Geometry check sheet. Reference: the model listing, model coordinates, mm. A direction names the side the tool comes from. Give positions to 0.01 mm unless a question says otherwise; leave off trailing zeros. Write each loop counter-clockwise with the first axis right and the second up, starting at its lowest first coordinate (ties: lowest second). Pieces come first, ordered by that corner, then holes. Notation, with made-up numbers: M 39,41.25 L 87,41.25 A19 ccw 87,77.25 Z; hole C 58.5,49.25 d9. An arc over 180 degrees is marked long. Use one line per item in the form item = value. Start each with the question number.
```python
from build123d import *

# Parameters (mm, degrees)
SKETCH1_W           = 22
SKETCH1_H           = 22
BOSS_EXTRUDE1_DEPTH = 17
SKETCH5_R           = 7
BOSS_EXTRUDE4_DEPTH = 3
SKETCH6_R           = 10
BOSS_EXTRUDE5_DEPTH = 13
SKETCH7_R           = 5.5
CUT_EXTRUDE1_DEPTH  = 37.482872694
SKETCH8_R           = 3.25
CUT_EXTRUDE2_DEPTH  = 46.5


with BuildPart() as part:
    # Sketch1 → Boss-Extrude1 (new body)
    with BuildSketch(Plane.XY):
        Rectangle(SKETCH1_W, SKETCH1_H)
    extrude(amount=BOSS_EXTRUDE1_DEPTH)

    # Sketch5 → Boss-Extrude4 (add)
    with BuildSketch(Plane.XY):
        Circle(SKETCH5_R)
    extrude(amount=-BOSS_EXTRUDE4_DEPTH)

    # Sketch6 → Boss-Extrude5 (add)
    with BuildSketch(Plane(origin=(0, 0, -3), x_dir=(-1, 0, 0), z_dir=(0, 0, -1))):
        Circle(SKETCH6_R)
    extrude(amount=BOSS_EXTRUDE5_DEPTH)

    # Sketch7 → Cut-Extrude1 (cut, through all)
    with BuildSketch(Plane.XY.offset(17)):
        Circle(SKETCH7_R)
    extrude(amount=-CUT_EXTRUDE1_DEPTH, mode=Mode.SUBTRACT)

    # Sketch8 → Cut-Extrude2 (cut, symmetric)
    with BuildSketch(Plane(origin=(11, 0, 0), x_dir=(0, 0, -1), z_dir=(1, 0, 0))):
        with Locations(Location((-8.5, 0, 0), (0, 0, 90))):
            Circle(SKETCH8_R)
    extrude(amount=CUT_EXTRUDE2_DEPTH, both=True, mode=Mode.SUBTRACT)


solid = part.part
```
(1) Sectioned sample at A-A, the plane x = 0. Record the boundary of the cut face in (y, z), plus the area to 3 significant figures.
(2) Sectioned sample at B-B, the plane z = 8.5. Record the boundary of the cut face in (x, y).
(3) Tool access check on faces 5 (the cylindrical face through (2.17, -9.76, -9.41)), 6 (the cylindrical face through (6.466, -2.681, -1.479)), 7 (the flat face through (11, -3, 6)). Record the directions out of +Z, -Z, +X, -X, +Y, -Y that give a thin tool (end or side, any length) a straight path to the whole face; none if there is none.
(4) Sectioned sample at C-C, the plane y = 0. Record the boundary of the cut face in (x, z).
(5) Depth check by flat-ended pin: pin 1 (4 mm diameter, centred on y = -3, z = -5, fed in from -X); pin 2 (5 mm diameter, centred on x = 6, z = -5, fed in from +Y); pin 3 (10 mm diameter, centred on y = 1, z = -5.5, fed in from -X). Enter the tip coordinate at first touch or a pass-through.
(6) Thickness scan on probe 1 along Z at (x, y) = (-7.5, 0); probe 2 along Y at (x, z) = (8.75, 8.5); probe 3 along Z at (x, y) = (6, -7.75). Record the ranges inside material, lowest first. Write a range as [from, to].
(7) Draft check along Y on faces 1 (the cylindrical face through (7.76, 3.1, 9.48)), 2 (the flat face through (-5, 3, 17)), 3 (the cylindrical face through (-7.67, 3.1, 9.48)), 4 (the flat face through (0, -11, 8)). Enter one of: released by +Y, released by -Y, zero draft, split by the parting line, or undercut.
(8) Sectioned sample at D-D, the plane x = -8.5. Record the boundary of the cut face in (y, z), plus the area to 3 significant figures.
Numbers:
q1.outline = M -11,0 L -7,0 L -7,-3 L -10,-3 L -10,-16 L -5.5,-16 L -5.5,17 L -11,17 Z; M 5.5,-16 L 10,-16 L 10,-3 L 7,-3 L 7,0 L 11,0 L 11,17 L 5.5,17 Z
q1.area = 313 mm2
q2.outline = M -11,-11 L 11,-11 L 11,-3.25 L 4.44,-3.25 A5.5 cw -4.44,-3.25 L -11,-3.25 Z; M -11,3.25 L -4.44,3.25 A5.5 cw 4.44,3.25 L 11,3.25 L 11,11 L -11,11 Z
q3.face_5 = -Z
q3.face_6 = none
q3.face_7 = +Z, -Z, +X, +Y, -Y
q4.outline = M -11,0 L -7,0 L -7,-3 L -10,-3 L -10,-16 L -5.5,-16 L -5.5,5.25 L -11,5.25 Z; M -11,11.75 L -5.5,11.75 L -5.5,17 L -11,17 Z; M 5.5,-16 L 10,-16 L 10,-3 L 7,-3 L 7,0 L 11,0 L 11,5.25 L 5.5,5.25 Z; M 5.5,11.75 L 11,11.75 L 11,17 L 5.5,17 Z
q5.pin_1 = -9.95
q5.pin_2 = 9.37
q5.pin_3 = -10
q6.probe_1 = [-16, -3], [0, 5.25], [11.75, 17]
q6.probe_2 = [-11, -3.25], [3.25, 11]
q6.probe_3 = [-16, -3], [0, 17]
q7.face_1 = undercut
q7.face_2 = zero draft
q7.face_3 = undercut
q7.face_4 = released by -Y
q8.outline = M -11,0 L 11,0 L 11,17 L -11,17 Z; M -5.27,-16 L 5.27,-16 L 5.27,-3 L -5.27,-3 Z; hole C 0,8.5 d6.5
q8.area = 478 mm2
